```python
from build123d import *

# Parameters (mm, degrees)
CROQUIS1_W              = 20
CROQUIS1_H              = 20
SALIENTE_EXTRUIR1_DEPTH = 300
CORTAR_EXTRUIR1_DEPTH   = 320


with BuildPart() as part:
    # Croquis1 → Saliente-Extruir1 (new body)
    with BuildSketch(Plane.XY):
        with Locations((-13.532555049, 4.541666667)):
            Rectangle(CROQUIS1_W, CROQUIS1_H)
    extrude(amount=SALIENTE_EXTRUIR1_DEPTH)

    # Croquis2 → Cortar-Extruir1 (cut)
    with BuildSketch(Plane.XY.offset(300)):
        Polygon((-13.532555049, 9.541666667), (-17.532555049, 9.541666667), (-17.532555049, 14.541666667), (-9.532555049, 14.541666667), (-9.532555049, 9.541666667), align=None)
        Polygon((-9.532555049, -0.458333333), (-9.532555049, -5.458333333), (-17.532555049, -5.458333333), (-17.532555049, -0.458333333), (-13.532555049, -0.458333333), align=None)
        Polygon((-23.532555049, 4.541666667), (-23.532555049, 8.541666667), (-18.532555049, 8.541666667), (-18.532555049, 0.541666667), (-23.532555049, 0.541666667), align=None)
        Polygon((-8.532555049, 8.541666667), (-8.532555049, 0.541666667), (-3.532555049, 0.541666667), (-3.532555049, 4.541666667), (-3.532555049, 8.541666667), align=None)
    extrude(amount=-CORTAR_EXTRUIR1_DEPTH, mode=Mode.SUBTRACT)


solid = part.part
```
Build history of the part. All positions in model axes, mm. A direction names the side the tool comes from. Give positions to 0.01 mm unless a question says otherwise; leave off trailing zeros. Loops run counter-clockwise (first coordinate to the right, second up) from the corner with the lowest first, then second, coordinate; pieces in that order, holes last. Notation, with made-up numbers: (41, 50) - (72, 50) arc R16 cw to (72, 62) - close; hole circle Ø7 at (18, 70.25). An arc over 180 degrees is marked (long way). Use a Markdown table: item, result.
(1) Wall check: line 1 along X through (y, z) = (11.75, 172); line 2 along Y through (x, z) = (-18.75, 268); line 3 along X through (y, z) = (1.25, 112.5). Give the ranges that are in metal, low to high.
Taken from the geometry:
| item | result |
|---|---|
| line 1 | -23.53 to -17.53, -9.53 to -3.53 |
| line 2 | -5.46 to 0.54, 8.54 to 14.54 |
| line 3 | -18.53 to -8.53 |
(2) Band-saw the part on A-A (y = -3). Give the cut face in (x, z).
Taken from the geometry:
| item | result |
|---|---|
| outline | (-23.53, 0) - (-17.53, 0) - (-17.53, 300) - (-23.53, 300) - close; (-9.53, 0) - (-3.53, 0) - (-3.53, 300) - (-9.53, 300) - close |
(3) Pull direction Y, two halves, no side cores. Call faces 4 (the face through (-6, 0.542, 152)), 5 (the face through (-23.533, -3, 148)), 6 (the face through (-7, -5.458, 148)): +Y half, -Y half, draft (parallel to the pull), parting line (faces both ways), or undercut.
Taken from the geometry:
| item | result |
|---|---|
| face 4 | undercut |
| face 5 | draft |
| face 6 | -Y half |
(4) Drop a flat-ended pin along its axis: pin 1 Ø6 at (x, y) = (-10.5, 12) entering from +Z. Give the stop position or say it passes through.
Taken from the geometry:
| item | result |
|---|---|
| pin 1 | z = 300 |
(5) Band-saw the part on C-C (x = -14.25). Give the cut face in (y, z).
Taken from the geometry:
| item | result |
|---|---|
| outline | (-0.46, 0) - (9.54, 0) - (9.54, 300) - (-0.46, 300) - close |
(6) Band-saw the part on B-B (z = 270). Give the cut face in (x, y).
Taken from the geometry:
| item | result |
|---|---|
| outline | (-23.53, -5.46) - (-17.53, -5.46) - (-17.53, -0.46) - (-9.53, -0.46) - (-9.53, -5.46) - (-3.53, -5.46) - (-3.53, 0.54) - (-8.53, 0.54) - (-8.53, 8.54) - (-3.53, 8.54) - (-3.53, 14.54) - (-9.53, 14.54) - (-9.53, 9.54) - (-17.53, 9.54) - (-17.53, 14.54) - (-23.53, 14.54) - (-23.53, 8.54) - (-18.53, 8.54) - (-18.53, 0.54) - (-23.53, 0.54) - close |
(7) Which spindle directions (+Z, -Z, +X, -X, +Y, -Y) get a long thin tool onto all of the face, cutting with end or side? Do faces 1 (the face through (-17.533, 12, 152)), 2 (the face through (-8.533, 5, 152)), 3 (the face through (-21, 0.542, 152)). Say none if no direction does.
Taken from the geometry:
| item | result |
|---|---|
| face 1 | +Z, -Z, +Y |
| face 2 | +Z, -Z, +X |
| face 3 | +Z, -Z, -X |
